The listing builds one solid part. Answer for the finished solid, in the listing's coordinates (mm). A direction names the side the tool comes from. Coordinates: 2 decimals unless noted, no trailing zeros. Write each loop counter-clockwise with the first axis right and the second up, starting at its lowest first coordinate (ties: lowest second). Pieces come first, ordered by that corner, then holes.
from build123d import *

# Parameters (mm, degrees)
BASE_FLANGE1_DEPTH            = 1
EDGE_FLANGE1_STRIP_W          = 5.4732
EDGE_FLANGE1_STRIP_H          = 1
EDGE_FLANGE1_STRIP_CUT_DEPTH  = 100
EDGE_FLANGE1_RELIEF_W         = 5.9732
EDGE_FLANGE1_RELIEF_H         = 0.5
EDGE_FLANGE1_RELIEF_CUT_DEPTH = 1
EDGE_FLANGE1_DEPTH            = 100
EDGE_FLANGE1_PROFILE_W        = 100
EDGE_FLANGE1_PROFILE_H        = 19.2634
EDGE_FLANGE1_PROFILE_R        = 1.5
EDGE_FLANGE1_FLAT_DEPTH       = 1
EDGE_FLANGE2_START            = -132.311951656
EDGE_FLANGE2_DEPTH            = 61
EDGE_FLANGE2_2_DEPTH          = 0.5
EDGE_FLANGE2_START_2          = -71.811951656
EDGE_FLANGE2_3_DEPTH          = 0.5
EDGE_FLANGE2_START_3          = -131.811951656
EDGE_FLANGE2_4_DEPTH          = 60
EDGE_FLANGE2_START_4          = -321.467617465
EDGE_FLANGE2_5_OUTLINE_R      = 1.5
EDGE_FLANGE2_5_DEPTH          = 1.000000001


with BuildPart() as part:
    # Base-Flange1: sheet metal written as solids
    # Sketch1 → Base-Flange1 (new body)
    with BuildSketch(Plane(origin=(0, 0, 0), x_dir=(0, 0, -1), z_dir=(1, 0, 0))):
        with BuildLine():
            Line((-292.608082875, 184.688048344), (277.391917125, 118.188048344))
            Line((277.391917125, 118.188048344), (277.391917125, -161.811951656))
            Line((277.391917125, -161.811951656), (-322.608082875, -161.811951656))
            Line((-322.608082875, -161.811951656), (-322.608082875, 188.188048344))
            Line((-322.608082875, 188.188048344), (-322.608082875, 213.188048344))
            ThreePointArc((-322.608082875, 213.188048344), (-332.239042701, 199.181856584), (-348.764537222, 203.161407511))
            ThreePointArc((-348.764537222, 203.161407511), (-336.339280516, 254.75856393), (-292.608082875, 224.688048344))
            Line((-292.608082875, 224.688048344), (-292.608082875, 184.688048344))
        make_face()
    extrude(amount=-BASE_FLANGE1_DEPTH)

    # Edge-Flange1: sheet metal written as solids
    # Edge-Flange1 strip (on a plane across the edge) → Edge-Flange1 strip cut (cut)
    with BuildSketch(Plane(origin=(-1, -161.811951656, -227.391917125), x_dir=(0, 1, 0), z_dir=(0, 0, 1))):
        with Locations((-1, -0.5)):
            Rectangle(EDGE_FLANGE1_STRIP_W, EDGE_FLANGE1_STRIP_H)
    edge_flange1_strip_cut = extrude(amount=EDGE_FLANGE1_STRIP_CUT_DEPTH, mode=Mode.SUBTRACT)

    # Edge-Flange1 relief (on the sheet) → Edge-Flange1 relief cut (cut)
    with BuildSketch(Plane(origin=(-1, -160.075351656, -227.391917125), x_dir=(0, 1, 0), z_dir=(-1, 0, 0))):
        with Locations((-2.4866, 0.25)):
            Rectangle(EDGE_FLANGE1_RELIEF_W, EDGE_FLANGE1_RELIEF_H)
        with Locations((-2.4866, -100.25)):
            Rectangle(EDGE_FLANGE1_RELIEF_W, EDGE_FLANGE1_RELIEF_H)
    edge_flange1_relief_cut = extrude(amount=-EDGE_FLANGE1_RELIEF_CUT_DEPTH, mode=Mode.SUBTRACT)

    # Edge-Flange1 bend section (on a plane across the edge) → Edge-Flange1 (add)
    with BuildSketch(Plane(origin=(-1, -161.811951656, -227.391917125), x_dir=(0, 1, 0), z_dir=(0, 0, 1))):
        with BuildLine():
            Line((0, 0.7366), (1, 0.7366))
            ThreePointArc((1, 0.7366), (1.215745145, 0.215745145), (1.7366, 0))
            Line((1.7366, 0), (1.7366, -1))
            ThreePointArc((1.7366, -1), (0.508638364, -0.491361636), (0, 0.7366))
        make_face()
    edge_flange1 = extrude(amount=EDGE_FLANGE1_DEPTH)

    # Edge-Flange1 profile (on flange) → Edge-Flange1 flat (add)
    with BuildSketch(Plane(origin=(-1, -161.811951656, 0), x_dir=(0, 0, -1), z_dir=(0, 1, 0))):
        with Locations((177.391917125, 10.3683)):
            Rectangle(EDGE_FLANGE1_PROFILE_W, EDGE_FLANGE1_PROFILE_H)
        with Locations((142.391917125, 10)):
            Circle(EDGE_FLANGE1_PROFILE_R, mode=Mode.SUBTRACT)
        with Locations((212.391917125, 10)):
            Circle(EDGE_FLANGE1_PROFILE_R, mode=Mode.SUBTRACT)
        with Locations((177.391917125, 10)):
            Circle(EDGE_FLANGE1_PROFILE_R, mode=Mode.SUBTRACT)
    edge_flange1_flat = extrude(amount=EDGE_FLANGE1_FLAT_DEPTH)

    # Mirror1: Edge-Flange1 strip cut, Edge-Flange1 relief cut, Edge-Flange1, Edge-Flange1 flat across plane
    add(edge_flange1_strip_cut.mirror(Plane.XY), mode=Mode.SUBTRACT)
    add(edge_flange1_relief_cut.mirror(Plane.XY), mode=Mode.SUBTRACT)
    add(edge_flange1.mirror(Plane.XY))
    add(edge_flange1_flat.mirror(Plane.XY))

    # Edge-Flange2: read off the stored shape, not the designer's step
    # Edge-Flange2 outline → Edge-Flange2 (cut)
    with BuildSketch(Plane(origin=(0, 0, 0), x_dir=(1, 0, 0), z_dir=(0, 1, 0)).offset(EDGE_FLANGE2_START)):
        with BuildLine():
            Line((0, -322.608082875), (0, -320.800405196))
            ThreePointArc((0, -320.800405196), (-0.271171885, -321.73223136), (-1, -322.373046287))
            Line((-1, -322.373046287), (-1, -322.608082875))
            Line((-1, -322.608082875), (0, -322.608082875))
        make_face()
    edge_flange2 = extrude(amount=EDGE_FLANGE2_DEPTH, mode=Mode.SUBTRACT)

    # Edge-Flange2 2 outline → Edge-Flange2 2 (cut)
    with BuildSketch(Plane(origin=(0, 0, 0), x_dir=(1, 0, 0), z_dir=(0, 1, 0)).offset(EDGE_FLANGE2_START)):
        with BuildLine():
            Line((0, -320.300405196), (-1, -320.300405196))
            Line((-1, -320.300405196), (-1, -322.373046287))
            ThreePointArc((-1, -322.373046287), (-0.271171885, -321.73223136), (0, -320.800405196))
            Line((0, -320.800405196), (0, -320.300405196))
        make_face()
    edge_flange2_2 = extrude(amount=EDGE_FLANGE2_2_DEPTH, mode=Mode.SUBTRACT)

    # Edge-Flange2 3 outline → Edge-Flange2 3 (cut)
    with BuildSketch(Plane(origin=(0, 0, 0), x_dir=(1, 0, 0), z_dir=(0, 1, 0)).offset(EDGE_FLANGE2_START_2)):
        with BuildLine():
            Line((0, -320.300405196), (-1, -320.300405196))
            Line((-1, -320.300405196), (-1, -322.373046287))
            ThreePointArc((-1, -322.373046287), (-0.271171885, -321.73223136), (0, -320.800405196))
            Line((0, -320.800405196), (0, -320.300405196))
        make_face()
    edge_flange2_3 = extrude(amount=EDGE_FLANGE2_3_DEPTH, mode=Mode.SUBTRACT)

    # Edge-Flange2 4 outline → Edge-Flange2 4 (add)
    with BuildSketch(Plane(origin=(0, 0, 0), x_dir=(1, 0, 0), z_dir=(0, 1, 0)).offset(EDGE_FLANGE2_START_3)):
        with BuildLine():
            Line((-1, -322.373046287), (-1, -320.800405196))
            ThreePointArc((-1, -320.800405196), (-1.238960253, -321.343483682), (-1.80079892, -321.53420221))
            Line((-1.80079892, -321.53420221), (-20.923893962, -319.861148183))
            Line((-20.923893962, -319.861148183), (-21.011049705, -320.857342881))
            Line((-21.011049705, -320.857342881), (-1.887954663, -322.530396908))
            ThreePointArc((-1.887954663, -322.530396908), (-1.433585428, -322.510364765), (-1, -322.373046287))
        make_face()
    edge_flange2_4 = extrude(amount=EDGE_FLANGE2_4_DEPTH)

    # Edge-Flange2 5 outline → Edge-Flange2 5 (cut)
    with BuildSketch(Plane(origin=(0, 0, 0), x_dir=(0.9961946980917458, 0, 0.0871557427476548), z_dir=(0.0871557427476548, 0, -0.9961946980917459)).offset(EDGE_FLANGE2_START_4)):
        with Locations((17.033463718, 121.811951656)):
            Circle(EDGE_FLANGE2_5_OUTLINE_R)
        with Locations((17.033463718, 101.811951656)):
            Circle(EDGE_FLANGE2_5_OUTLINE_R)
        with Locations((17.033463718, 81.811951656)):
            Circle(EDGE_FLANGE2_5_OUTLINE_R)
    edge_flange2_5 = extrude(amount=EDGE_FLANGE2_5_DEPTH, mode=Mode.SUBTRACT)

    # Mirror2: Edge-Flange2, Edge-Flange2 2, Edge-Flange2 3, Edge-Flange2 4, Edge-Flange2 5 across plane
    add(edge_flange2.mirror(Plane.ZX), mode=Mode.SUBTRACT)
    add(edge_flange2_2.mirror(Plane.ZX), mode=Mode.SUBTRACT)
    add(edge_flange2_3.mirror(Plane.ZX), mode=Mode.SUBTRACT)
    add(edge_flange2_4.mirror(Plane.ZX))
    add(edge_flange2_5.mirror(Plane.ZX), mode=Mode.SUBTRACT)


solid = part.part
Q1. The part is cut by section B-B, the plane y = 191. Write down the section's boundary in (x, z).
Answers below:
outline: (-1, 292.61) - (0, 292.61) - (0, 322.61) - (-1, 322.61) - close
Q2. The part is cut by section C-C, the plane z = -195.5. Write down the section's boundary in (x, y), then the cut area to 3 significant figures.
Answers below:
outline: (-21, -161.81) - (-1.74, -161.81) arc R1.74 ccw to (0, -160.08) - (0, 127.74) - (-1, 127.74) - (-1, -160.08) arc R0.74 cw to (-1.74, -160.81) - (-21, -160.81) - close
area: 309 mm2
Q3. The part is cut by section A-A, the plane x = -5.5. Write down the section's boundary in (y, z), then the cut area to 3 significant figures.
Answers below:
outline: (-161.81, -227.39) - (-160.81, -227.39) - (-160.81, -127.39) - (-161.81, -127.39) - close; (-161.81, 127.39) - (-160.81, 127.39) - (-160.81, 227.39) - (-161.81, 227.39) - close; (-131.81, 321.21) - (-71.81, 321.21) - (-71.81, 322.21) - (-131.81, 322.21) - close; (71.81, 321.21) - (131.81, 321.21) - (131.81, 322.21) - (71.81, 322.21) - close
area: 320 mm2
Q4. Find the intervals of material crossed by probe 1 along X at (y, z) = (30.5, 128.5); probe 2 along Y at (x, z) = (-2.5, 136.5); probe 3 along Z at (x, y) = (-20, -116), in increasing order.
Answers below:
probe 1: x = -1 to 0
probe 2: y = -161.81 to -160.81
probe 3: z = 319.94 to 320.95
Q5. Determine the mould class of faces 4 (the face through (-0.493, 199.274, 332.004)), 5 (the face through (-9.104, 102.232, 320.895)), 6 (the face through (-14, -160.812, 177)) for opening direction Z: released by +Z, released by -Z, zero draft, split by the parting line, or undercut.
Answers below:
face 4: undercut
face 5: released by -Z
face 6: zero draft
Q6. Given pin 1 (0.7 mm diameter, centred on x = -7, y = -161, fed in from +Z); pin 2 (8 mm diameter, centred on y = 33, z = 15, fed in from -X); pin 3 (1.1 mm diameter, centred on x = -0.5, z = 321, fed in from +Y), each flat-ended and moving along its own axis, determine where each tip first touches the part or whether it passes through.
Answers below:
pin 1: stops at z = 227.39
pin 2: stops at x = -1
pin 3: stops at y = 256.73
Q7. Which of the six approach directions +Z, -Z, +X, -X, +Y, -Y give full straight-line access (tool end or side, diameter ignored) to faces 1 (the face through (-9.104, -102.232, 320.895)), 2 (the face through (-14, -160.812, -177)), 3 (the face through (-14, -161.812, -177))?
Answers below:
face 1: -Z, +Y, -Y
face 2: +Z, -Z, -X, +Y
face 3: +Z, -Z, +X, -X, -Y
